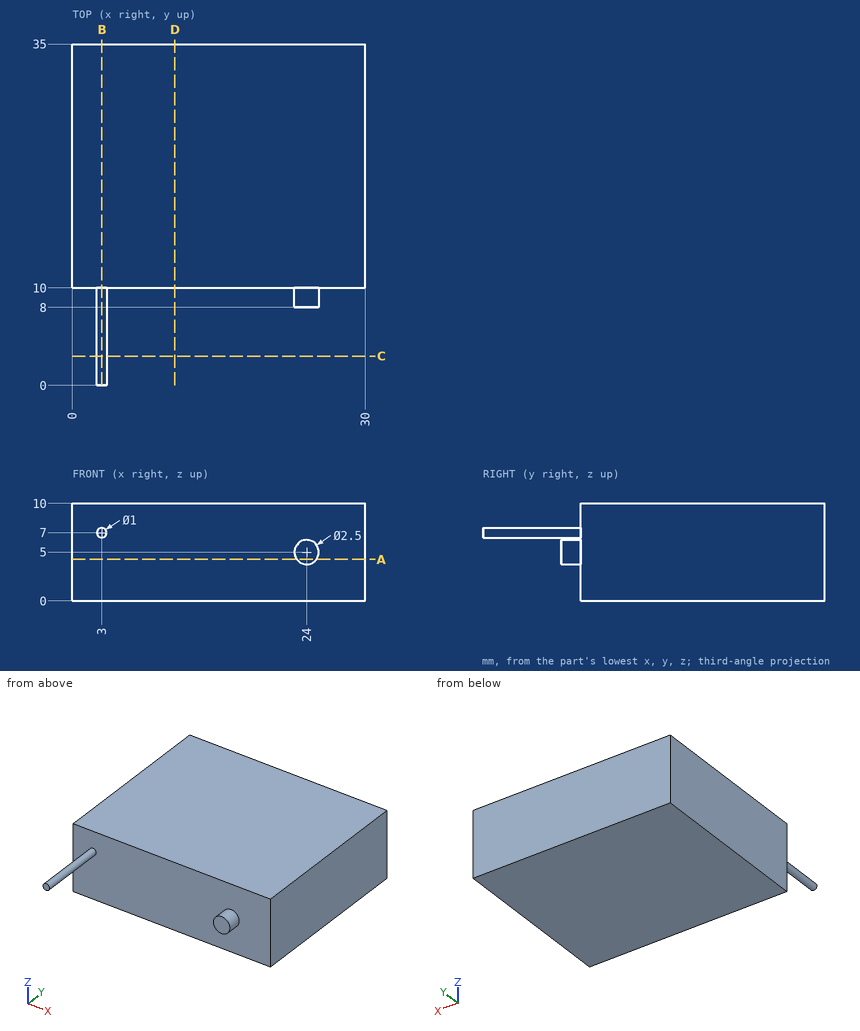
Here's the drawing with two shaded views (mm, measured from the low corner). I have some questions. Give positions to 0.01 mm unless a question says otherwise; leave off trailing zeros. Loops run counter-clockwise (first coordinate to the right, second up) from the corner with the lowest first, then second, coordinate; pieces in that order, holes last. Notation, with made-up numbers: (63, 17.5) -> (108, 17.5) arc R24 cw to (108, 54.5) -> close; hole circle Ø4 at (48.25, 31.5). An arc over 180 degrees is marked (long way). One line per item, written item: value.
Q1. If I drill on line 1 along Y through (x, z) = (21.5, 6); line 2 along X through (y, z) = (3, 6.75), over which ranges is the centre line in solid material (lowest first)?
Answers follow:
line 1: 10 to 35
line 2: 2.57 to 3.43
Q2. I'm going to push flat-ended pins straight in: pin 1 Ø6 at (y, z) = (18.5, 6) entering from -X; pin 2 Ø3 at (x, z) = (24.5, 4.5) entering from -Y; pin 3 Ø3 at (x, z) = (7.5, 5) entering from -Y. Where does each tip first touch, or does it pass through?
Answers follow:
pin 1: x = 0
pin 2: y = 8
pin 3: y = 10
Q3. Suppose I cut it at C-C on y = 3. Please give me the cut outline in (x, z), then the cut area to 3 significant figures.
Answers follow:
outline: circle Ø1 at (3, 7)
area: 0.785 mm^2
Q4. Suppose I cut it at A-A on z = 4.25. Please give me the cut outline in (x, y).
Answers follow:
outline: (0, 10) -> (23, 10) -> (23, 8) -> (25, 8) -> (25, 10) -> (30, 10) -> (30, 35) -> (0, 35) -> close
Q5. Suppose I cut it at B-B on x = 3. Please give me the cut outline in (y, z).
Answers follow:
outline: (0, 6.5) -> (10, 6.5) -> (10, 0) -> (35, 0) -> (35, 10) -> (10, 10) -> (10, 7.5) -> (0, 7.5) -> close
Q6. Suppose I cut it at D-D on x = 10.5. Please give me the cut outline in (y, z).
Answers follow:
outline: (10, 0) -> (35, 0) -> (35, 10) -> (10, 10) -> close
